Answer from the drawing. Dimensions are ordinates in mm from the lowest x, y and z of the part. Coordinates: 2 decimals unless noted, no trailing zeros. Write each loop counter-clockwise with the first axis right and the second up, starting at its lowest first coordinate (ties: lowest second). Pieces come first, ordered by that corner, then holes. Notation, with made-up numbers: (15.5, -8) -> (42.5, -8) arc R14 cw to (42.5, 11) -> close; hole circle Ø3 at (84.5, 1). An arc over 180 degrees is marked (long way). Answer as a JSON object with one key per item and string values. Group by question number.
(1) Find section D-D (x = 223). Give the vertices of the cut face in (y, z), then the cut area to 3 significant figures.
(2) Find section B-B (z = 351). Give the vertices of the cut face in (x, y), then the cut area to 3 significant figures.
(3) Straight lines are drawn through the part: L1, parallel to X at y = 8, z = 457; L2, parallel to Z at x = 160, y = 1.75; L3, parallel to Z at x = 385, y = 11.25. For each, find the intervals that lie inside material, in ascending order.
(4) Find section A-A (x = 550). Give the vertices of the cut face in (y, z).
(5) Find section C-C (y = 3). Give the vertices of the cut face in (x, z).
(6) For a pull along X with two mould halves and no side action, classify the marked faces 1 and 2 as +X half, -X half, draft (parallel to the pull), parting line (faces both ways), or undercut.
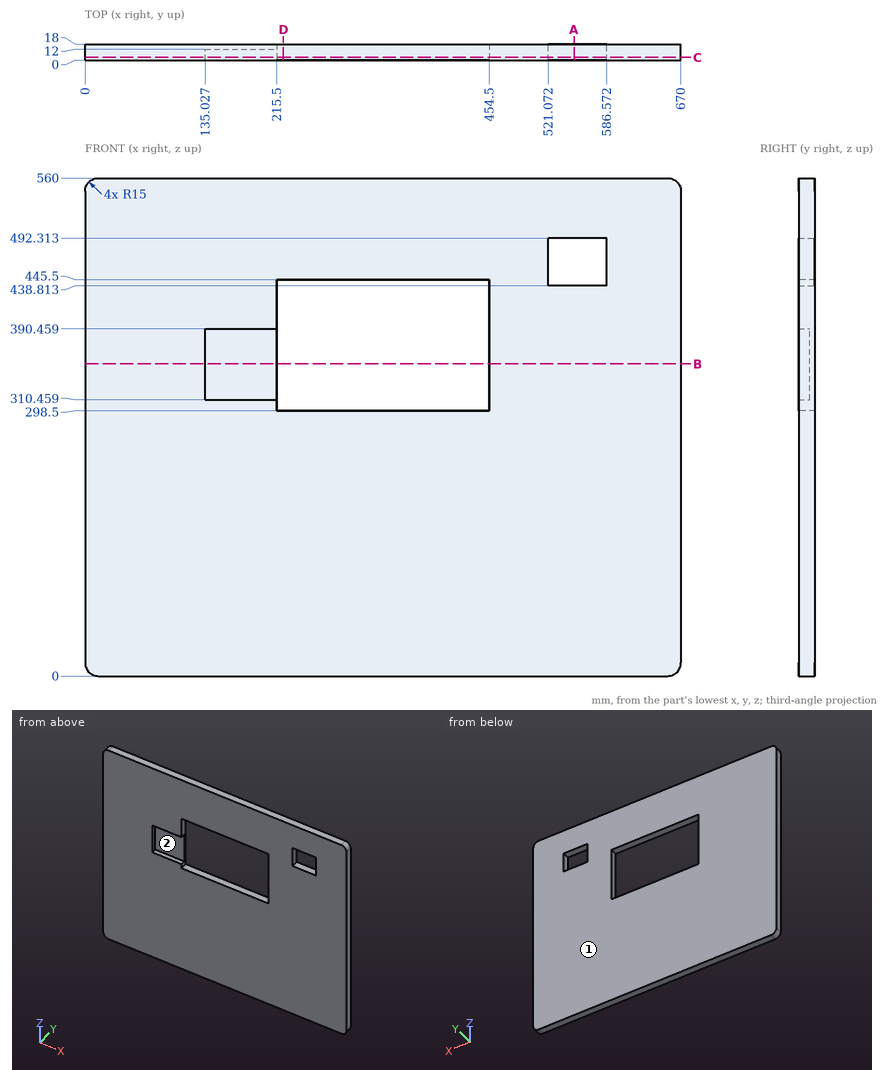
Results below:
{
 "1": {"outline": "(0, 0) -> (18, 0) -> (18, 298.5) -> (0, 298.5) -> close; (0, 445.5) -> (18, 445.5) -> (18, 560) -> (0, 560) -> close", "area": "7,430 mm2"},
 "2": {"outline": "(0, 0) -> (135.03, 0) -> (135.03, 12) -> (215.5, 12) -> (215.5, 18) -> (0, 18) -> close; (454.5, 0) -> (670, 0) -> (670, 18) -> (454.5, 18) -> close", "area": "6,790 mm2"},
 "3": {"L1": "x = 0 to 521.07, 586.57 to 670", "L2": "z = 0 to 310.46, 390.46 to 560", "L3": "z = 0 to 298.5, 445.5 to 560"},
 "4": {"outline": "(0, 0) -> (18, 0) -> (18, 438.81) -> (0, 438.81) -> close; (0, 492.31) -> (18, 492.31) -> (18, 560) -> (0, 560) -> close"},
 "5": {"outline": "(0, 15) arc R15 ccw to (15, 0) -> (655, 0) arc R15 ccw to (670, 15) -> (670, 545) arc R15 ccw to (655, 560) -> (15, 560) arc R15 ccw to (0, 545) -> close; hole (135.03, 310.46) -> (215.5, 310.46) -> (215.5, 298.5) -> (454.5, 298.5) -> (454.5, 445.5) -> (215.5, 445.5) -> (215.5, 390.46) -> (135.03, 390.46) -> close; hole (521.07, 438.81) -> (586.57, 438.81) -> (586.57, 492.31) -> (521.07, 492.31) -> close"},
 "6": {"face 1": "draft", "face 2": "undercut"}
}
